Job drawing, mm, ordinate dimensions from the low corner. One solid piece. A direction names the side the tool comes from. Give positions to 0.01 mm unless a question says otherwise; leave off trailing zeros. Order: outer loops, then holes, each group sorted by start corner. A loop starts at its lowest first (then second) coordinate and runs counter-clockwise, first axis right, second up. Notation, with made-up numbers: (21, 70) - (56, 70) arc R16 ccw to (56, 77) - close; hole circle Ø11 at (27.5, -10). An arc over 180 degrees is marked (long way). One line per item, written item: value.
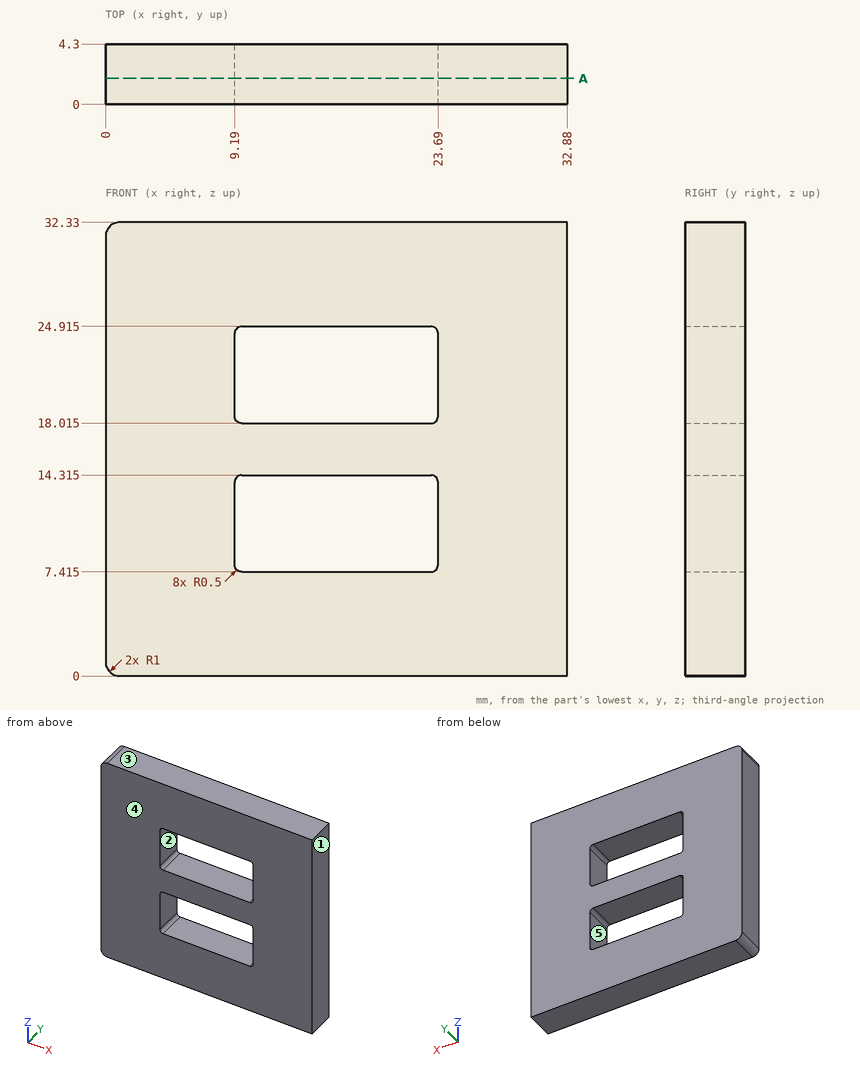
1) Two-plate mould, pull along Z, no slides. Class the marked faces 1, 2 and 3: pulls with the +Z half, pulls with the -Z half, needs draft (parallel to the pull), parting line crosses it, or undercut.
Answer:
face 1: needs draft
face 2: undercut
face 3: pulls with the +Z half
2) Wall check: line 1 along Z through (x, y) = (23, 2.15) (3 decimals); line 2 along X through (y, z) = (3.8, 8). Give the ranges that are in metal, low to high. Write a range as [from, to].
Answer:
line 1: z = [0, 7.415], [14.315, 18.015], [24.915, 32.33]
line 2: x = [0, 9.19], [23.69, 32.88]
3) Which spindle directions (+Z, -Z, +X, -X, +Y, -Y) get a long thin tool onto all of the face, cutting with end or side? Do the marked faces 4 and 5. Say none if no direction does.
Answer:
face 4: +Z, -Z, +X, -X, -Y
face 5: +Y, -Y
4) Slice it at A-A on y = 1.85. Write the cut outline in (x, z) (3 decimals).
Answer:
outline: (0, 1) arc R1 ccw to (1, 0) - (32.88, 0) - (32.88, 32.33) - (1, 32.33) arc R1 ccw to (0, 31.33) - close; hole (9.19, 7.915) arc R0.5 ccw to (9.69, 7.415) - (23.19, 7.415) arc R0.5 ccw to (23.69, 7.915) - (23.69, 13.815) arc R0.5 ccw to (23.19, 14.315) - (9.69, 14.315) arc R0.5 ccw to (9.19, 13.815) - close; hole (9.19, 18.515) arc R0.5 ccw to (9.69, 18.015) - (23.19, 18.015) arc R0.5 ccw to (23.69, 18.515) - (23.69, 24.415) arc R0.5 ccw to (23.19, 24.915) - (9.69, 24.915) arc R0.5 ccw to (9.19, 24.415) - close
